Build history of the part. All positions in model axes, mm. Face numbers are marked on the shaded views. Give positions to 0.01 mm unless a question says otherwise; leave off trailing zeros. Write each loop counter-clockwise with the first axis right and the second up, starting at its lowest first coordinate (ties: lowest second). Pieces come first, ordered by that corner, then holes. Notation, with made-up numbers: M -16.5,-8.5 L 1.5,-8.5 A26 cw 1.5,11.5 Z; hole C 32,51.5 d2. An arc over 180 degrees is marked long. One line per item, written item: value. Start each with the question number.
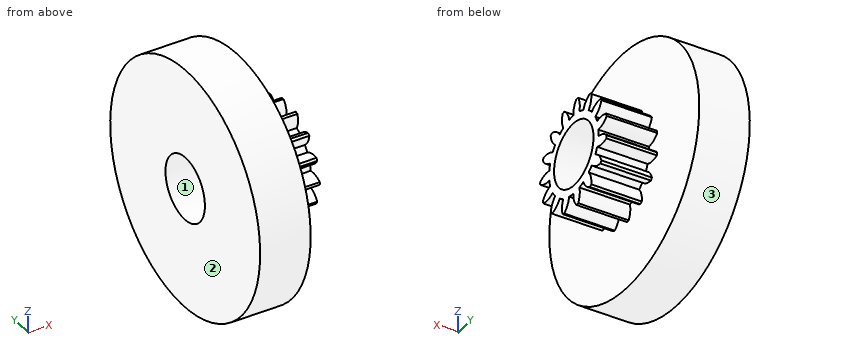
from build123d import *

# Parameters (mm, degrees)
BASPROSKE_W      = 4
BASPROSKE_H      = 4.25
TOOTHCUT_DEPTH   = 8.219764539
TEETHCUTS_COUNT  = 15
TEETHCUTS_ANGLE  = 336
HUBNEAONESKE_R   = 9.5
HUBNEARONE_DEPTH = 4.0001016
BORSKE_R         = 2.5
BORE_DEPTH       = 8.0001016


with BuildPart() as part:
    # BasProSke → Base-Revolve (revolve)
    with BuildSketch(Plane(origin=(0, 0, 0), x_dir=(1, 0, 0), z_dir=(0, 1, 0)), mode=Mode.PRIVATE) as base_revolve_sk:
        with Locations((2, 2.125)):
            Rectangle(BASPROSKE_W, BASPROSKE_H)
    revolve(base_revolve_sk.sketch.rotate(Axis((-10, 0, 0), (1, 0, 0)), 180), axis=Axis((-10, 0, 0), (1, 0, 0)))

    # TooCutSke → ToothCut (cut, through all)
    with BuildSketch(Plane(origin=(0, 0, 0), x_dir=(0, 0, -1), z_dir=(1, 0, 0))):
        with BuildLine():
            ThreePointArc((0.265767165, 3.112674704), (0, 3.124), (-0.265767165, 3.112674704))
            ThreePointArc((-0.265767165, 3.112674704), (-0.418628877, 3.712626775), (-0.800767345, 4.19974009))
            ThreePointArc((-0.800767345, 4.19974009), (0, 4.2754), (0.800767345, 4.19974009))
            ThreePointArc((0.800767345, 4.19974009), (0.418628877, 3.712626775), (0.265767165, 3.112674704))
        make_face()
    toothcut = extrude(amount=TOOTHCUT_DEPTH, mode=Mode.SUBTRACT)

    # TeethCuts: ToothCut ×15 about axis
    teethcuts_axis = Axis((-10, 0, 0), (1, 0, 0))
    for i in range(1, TEETHCUTS_COUNT):
        add(toothcut.rotate(teethcuts_axis, i * TEETHCUTS_ANGLE / (TEETHCUTS_COUNT - 1)), mode=Mode.SUBTRACT)

    # HubNeaOneSke → HubNearOne (add)
    with BuildSketch(Plane.ZY):
        Circle(HUBNEAONESKE_R)
    extrude(amount=HUBNEARONE_DEPTH)

    # BorSke → Bore (cut, symmetric)
    with BuildSketch(Plane(origin=(0, 0, 0), x_dir=(0, 0, -1), z_dir=(1, 0, 0))):
        with Locations(Location((0, 0, 0), (0, 0, 180))):
            Circle(BORSKE_R)
    extrude(amount=BORE_DEPTH, both=True, mode=Mode.SUBTRACT)


solid = part.part
1) Probe line 1 along Y through (x, z) = (-1, 0); line 2 along X through (y, z) = (-5.5, -1.25); line 3 along Y through (x, z) = (-0.5, -2.25). List the from-to ranges inside material, lowest first. Write a range as from..to.
2) Mould opens along Y. For the marked faces 1, 2 and 3 say: released by +Y, released by -Y, zero draft, split by the parting line, or undercut.
3) Drop flat-ended pins along their axis: P1, Ø1, axis at x = 2, z = -0.5, coming from the -Y side; P2, Ø1.5, axis at x = -2, z = -5.5, coming from the -Y side; P3, Ø4, axis at y = 0, z = 0, coming from the +X side; P4, Ø4, axis at x = -2.5, y = -5, coming from the -Z side. Give the stop position or say it passes through.
4) Band-saw the part on A-A (x = -1.5). List the corners of the cut face in (y, z).
5) Band-saw the part on B-B (z = -4.5). List the corners of the cut face in (x, y).
6) Band-saw the part on C-C (y = -6.5). List the corners of the cut face in (x, z).
Model answer:
1. line 1: y = -9.5..-2.5, 2.5..9.5
1. line 2: x = -4..0
1. line 3: y = -9.23..-1.09, 1.09..9.23
2. face 1: undercut
2. face 2: zero draft
2. face 3: split by the parting line
3. P1: stops at y = -4.25
3. P2: stops at y = -8.23
3. P3: passes through
3. P4: stops at z = -9.01
4. outline: C 0,0 d19; hole C 0,0 d5
5. outline: M -4,-8.37 L 0,-8.37 L 0,8.37 L -4,8.37 Z
6. outline: M -4,-6.93 L 0,-6.93 L 0,6.93 L -4,6.93 Z
